Geometry check sheet. Reference: the model listing, model coordinates, mm. Face numbers are marked on the shaded views. A direction names the side the tool comes from. Coordinates: 2 decimals unless noted, no trailing zeros. Write each loop counter-clockwise with the first axis right and the second up, starting at its lowest first coordinate (ties: lowest second). Pieces come first, ordered by that corner, then holes. Notation, with made-up numbers: M 70,35 L 121,35 A22 ccw 121,45 Z; hole C 51,-30.5 d1. An arc over 180 degrees is marked long. Write each question's results on one line, items separated by ' | '.
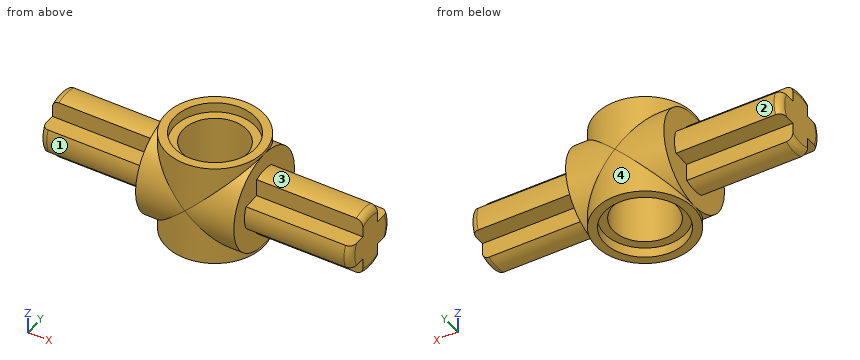
```python
from build123d import *

# Parameters (mm, degrees)
SKETCH1_W              = 1.8
SKETCH1_H              = 1.8
PIN_DEPTH              = 11.7
SKETCH2_R              = 3.7
MIDDLE_DEPTH           = 3.7
SKETCH6_R              = 3.7
MIDDLE_BODY_DEPTH      = 3.9
MIDDLE_BORE_DEPTH      = 13.875946567
MIDDLE_BORE_DEPTH_BACK = 13.875946567
SKETCH7_R              = 2.4
SKETCH8_R              = 3.05
MIDDLE_RIM_CUT_DEPTH   = 0.75
FILLET1_R              = 0.5


with BuildPart() as part:
    # Sketch1 → Pin (new, symmetric)
    with BuildSketch(Plane(origin=(0, 0, 0), x_dir=(0, 0, -1), z_dir=(1, 0, 0))):
        with BuildLine():
            Line((-0.9, 0.9), (0.9, 0.9))
            Line((0.9, 0.9), (0.9, 2.224859546))
            ThreePointArc((0.9, 2.224859546), (0.45844143, 2.355808026), (0, 2.4))
            ThreePointArc((0, 2.4), (-0.45844143, 2.355808026), (-0.9, 2.224859546))
            Line((-0.9, 2.224859546), (-0.9, 0.9))
        make_face()
        Rectangle(SKETCH1_W, SKETCH1_H)
        with BuildLine():
            Line((-2.224859546, -0.9), (-0.9, -0.9))
            Line((-0.9, -0.9), (-0.9, 0.9))
            Line((-0.9, 0.9), (-2.224859546, 0.9))
            ThreePointArc((-2.224859546, 0.9), (-2.355808027, 0.458441425), (-2.4, -1e-08))
            ThreePointArc((-2.4, -1e-08), (-2.355808025, -0.458441435), (-2.224859546, -0.9))
        make_face()
        with BuildLine():
            ThreePointArc((-0.9, -2.224859546), (-0.45844143, -2.355808026), (0, -2.4))
            ThreePointArc((0, -2.4), (0.45844143, -2.355808026), (0.9, -2.224859546))
            Line((0.9, -2.224859546), (0.9, -0.9))
            Line((0.9, -0.9), (-0.9, -0.9))
            Line((-0.9, -0.9), (-0.9, -2.224859546))
        make_face()
        with BuildLine():
            Line((0.9, 0.9), (0.9, -0.9))
            Line((0.9, -0.9), (2.224859546, -0.9))
            ThreePointArc((2.224859546, -0.9), (2.355808026, -0.45844143), (2.4, 0))
            ThreePointArc((2.4, 0), (2.355808026, 0.45844143), (2.224859546, 0.9))
            Line((2.224859546, 0.9), (0.9, 0.9))
        make_face()
    extrude(amount=PIN_DEPTH, both=True)

    # Sketch2 → Middle (add, symmetric)
    with BuildSketch(Plane(origin=(0, 0, 0), x_dir=(0, 0, -1), z_dir=(1, 0, 0))):
        Circle(SKETCH2_R)
    extrude(amount=MIDDLE_DEPTH, both=True)

    # Sketch6 → Middle Body (add, symmetric)
    with BuildSketch(Plane.XY):
        Circle(SKETCH6_R)
    extrude(amount=MIDDLE_BODY_DEPTH, both=True)

    # Sketch7 → Middle Bore (cut, two sides: drawn at the far end of the back side and taken through both)
    with BuildSketch(Plane.XY.offset(-MIDDLE_BORE_DEPTH_BACK)):
        Circle(SKETCH7_R)
    extrude(amount=MIDDLE_BORE_DEPTH + MIDDLE_BORE_DEPTH_BACK, mode=Mode.SUBTRACT)

    # Sketch8 → Middle Rim Cut (cut)
    with BuildSketch(Plane.XY.offset(3.9)):
        Circle(SKETCH8_R)
    middle_rim_cut = extrude(amount=-MIDDLE_RIM_CUT_DEPTH, mode=Mode.SUBTRACT)

    # Mirror2: Middle Rim Cut across plane
    add(middle_rim_cut.mirror(Plane.XY), mode=Mode.SUBTRACT)

    # Fillet1
    fillet1_edges = [part.edges().sort_by_distance(p)[0] for p in [
        (11.7, 2.4, 0),
        (-11.7, 0, -2.4),
        (-11.7, -2.4, 0),
        (-11.7, 0, 2.4),
        (-11.7, 2.4, 0),
        (11.7, 0, 2.4),
        (11.7, -2.4, 0),
        (11.7, 0, -2.4),
    ]]
    fillet(fillet1_edges, radius=FILLET1_R)


solid = part.part
```
Q1. Depth check by flat-ended pin: P1, Ø1, axis at x = -5, y = -1, coming from the -Z side; P2, Ø1.1, axis at x = 7, z = -1.5, coming from the +Y side; P3, Ø3.5, axis at x = 0, y = 0, coming from the -Z side; P4, Ø0.7, axis at x = -8, z = 2, coming from the -Y side. Enter the tip coordinate at first touch or a pass-through.
Geometry check:
P1: stops at z = -2.35 | P2: stops at y = 0.9 | P3: passes through | P4: stops at y = -0.9
Q2. Scan lines: probe 1 along Y at (x, z) = (0, 3.45); probe 2 along Y at (x, z) = (0, -1); probe 3 along X at (y, z) = (0, -0.5). Record each from-to range of solid material in increasing order.
Geometry check:
probe 1: y = -3.7 to -3.05, 3.05 to 3.7 | probe 2: y = -3.7 to -2.4, 2.4 to 3.7 | probe 3: x = -11.7 to -2.4, 2.4 to 11.7
Q3. Sectioned sample at B-B on x = -9.25. Record the cut outline in (y, z).
Geometry check:
outline: M -2.22,-0.9 L -0.9,-0.9 L -0.9,-2.22 A2.4 ccw 0.9,-2.22 L 0.9,-0.9 L 2.22,-0.9 A2.4 ccw 2.22,0.9 L 0.9,0.9 L 0.9,2.22 A2.4 ccw -0.9,2.22 L -0.9,0.9 L -2.22,0.9 A2.4 ccw Z
Q4. Access from +Z, -Z, +X, -X, +Y, -Y to the whole of each face (thin tool, end or side, straight path). Record for the marked faces 1, 2, 3 and 4.
Geometry check:
face 1: -X, -Y | face 2: -X, +Y | face 3: +Z, +X | face 4: -Z
